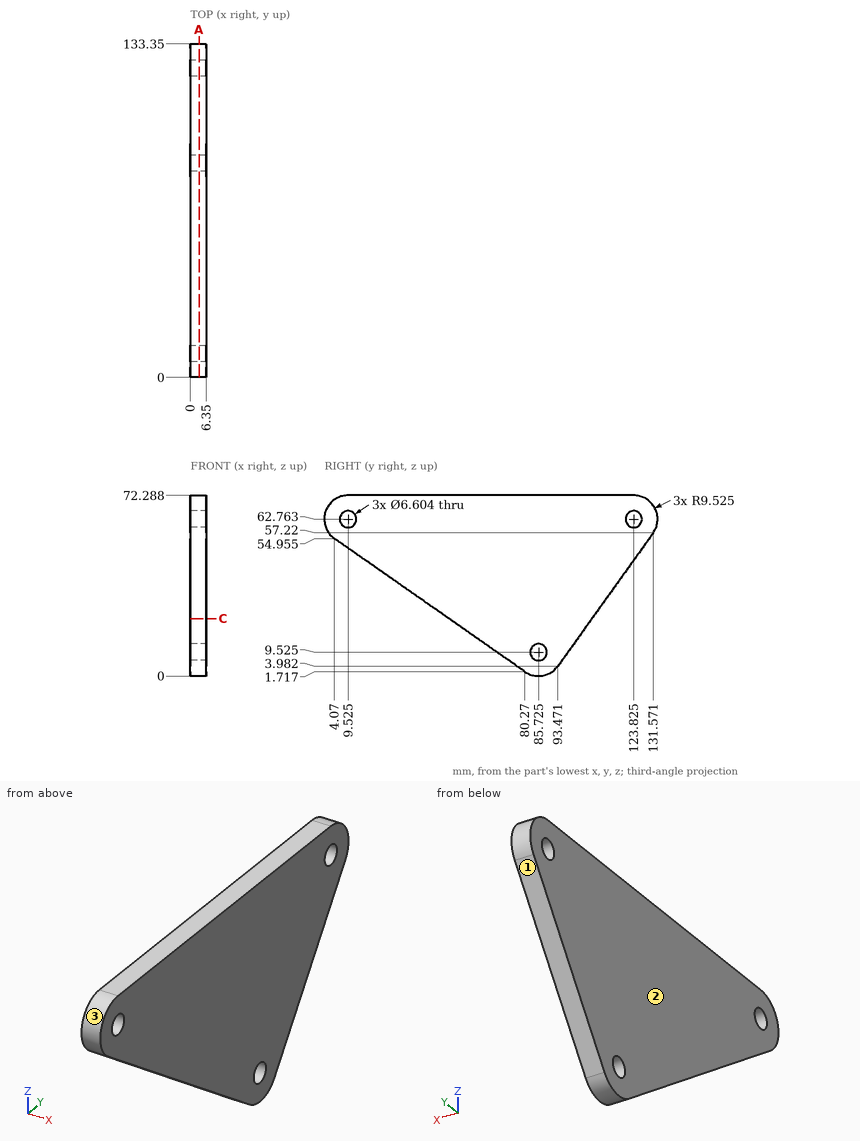
Here's the drawing with two shaded views (mm, measured from the low corner). I have some questions. Coordinates: 2 decimals unless noted, no trailing zeros. Write each loop counter-clockwise with the first axis right and the second up, starting at its lowest first coordinate (ties: lowest second). Pieces come first, ordered by that corner, then holes. Notation, with made-up numbers: (72, -25) - (90, -25) arc R28 cw to (90, -4) - close; hole circle Ø10 at (5, 6). An arc over 180 degrees is marked (long way). Return JSON: item names as keys, results as strings.
Q1. If we section it at A-A (x = 3.5): Count the separate pieces of the cut face and the enclosed holes in it, then the cut area to 3 significant figures.
Computed values:
{"separate pieces": "1", "enclosed holes": "3", "area": "5,820 mm2"}
Q2. I'm going to push flat-ended pins straight in: pin 1 Ø2 at (x, y) = (2, 88.5) entering from -Z; pin 2 Ø1 at (x, y) = (1, 15.5) entering from -Z; pin 3 Ø3 at (x, z) = (3.5, 30) entering from -Y. Where does each tip first touch, or does it pass through?
Computed values:
{"pin 1": "stops at z = 0.17", "pin 2": "stops at z = 46.62", "pin 3": "stops at y = 37.64"}
Q3. Thinking about a two-plate mould opening in Z: for the marked faces 1, 2 and 3, which applies, +Z half, -Z half, draft (parallel to the pull), parting line (faces both ways), or undercut?
Computed values:
{"face 1": "-Z half", "face 2": "draft", "face 3": "parting line"}
Q4. If we section it at C-C (z = 23): Please give me the cut outline in (x, y), then the cut area to 3 significant figures.
Computed values:
{"outline": "(0, 49.81) - (6.35, 49.81) - (6.35, 107.08) - (0, 107.08) - close", "area": "364 mm2"}
Q5. Please list where these lines run through material, in increasing order: L1, parallel to Y at x = 1.25, z = 60 (1 decimal); L2, parallel to Z at x = 2.25, y = 84; L3, parallel to Y at x = 1, z = 39 (1 decimal). Write a range as from..to.
Computed values:
{"L1": "y = 0.4..7.7, 11.3..122, 125.6..132.9", "L2": "z = 0.16..6.71, 12.34..72.29", "L3": "y = 26.9..118.5"}
